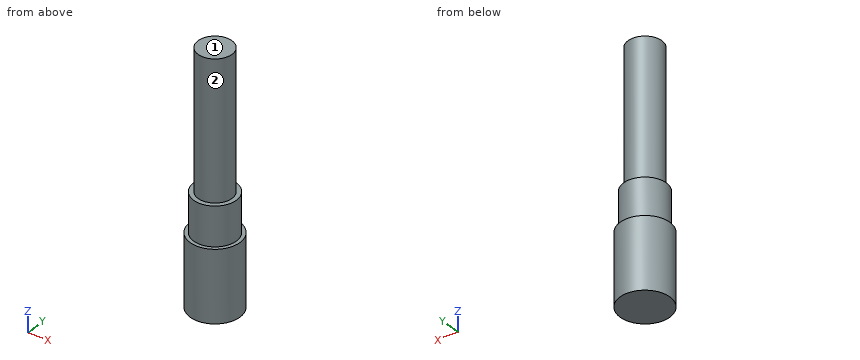
```python
from build123d import *

# Parameters (mm, degrees)
F0_R     = 15.38
F0_R_2   = 13.2
F1_DEPTH = 43.96
F0_R_3   = 10.45
F3_DEPTH = 68
F2_DEPTH = 152.8


with BuildPart() as f1:
    # F0 (on Top) → F1 (new body)
    with BuildSketch(Plane.XY):
        Circle(F0_R)
        Circle(F0_R_2, mode=Mode.SUBTRACT)
    extrude(amount=F1_DEPTH)

    # F0 (on Top) → F3 (join)
    with BuildSketch(Plane.XY):
        Circle(F0_R_2)
        Circle(F0_R_3, mode=Mode.SUBTRACT)
    extrude(amount=F3_DEPTH)

    # F0 (on Top) → F2 (join)
    with BuildSketch(Plane.XY):
        Circle(F0_R_3)
    extrude(amount=F2_DEPTH)


solid = f1.part
```
Geometry: final body of the model. Coordinates: model frame, mm. Face numbers are marked on the shaded views. A direction names the side the tool comes from. Round coordinates to 2 decimals unless told otherwise and drop trailing zeros. Order: outer loops, then holes, each group sorted by start corner. A loop starts at its lowest first (then second) coordinate and runs counter-clockwise, first axis right, second up. Notation, with made-up numbers: M 67.25,-16 L 125.25,-16 A21 cw 125.25,-3 Z; hole C -0.75,-16 d7. An arc over 180 degrees is marked long. Use one line per item in the form item = value. Start each with the question number.
Q1. Material intervals for line 1 (Z direction, x = 12.5, y = 7); line 2 (Z direction, x = -9, y = -8); line 3 (Y direction, x = 0.5, z = 86), sorted ascending. Write a range as [from, to].
Q2. Access query for the marked faces 1 and 2. Directions: +Z, -Z, +X, -X, +Y, -Y. A direction counts if a zero-diameter tool reaches every point of the face in a straight line with its end or side. Return the directions, or none.
Q3. Pin query (flat end, axial travel): pin 1 Ø1 at (y, z) = (9, 67) entering from -X; pin 2 Ø1 at (x, z) = (8, 98) entering from -Y; pin 3 Ø3 at (y, z) = (4.5, 123) entering from -X. Return the tip coordinate at first contact, or that it passes through.
Q4. Cut plane A-A (x = 0). Return loops of the section in (y, z).
Q5. Cut plane C-C (z = 125). Return loops of the section in (x, y).
Q6. Cut plane D-D (z = 19). Return loops of the section in (x, y), and give its area (3 significant figures).
Geometry results:
q1.line_1 = [0, 43.96]
q1.line_2 = [0, 68]
q1.line_3 = [-10.44, 10.44]
q2.face_1 = +Z, +X, -X, +Y, -Y
q2.face_2 = +Z
q3.pin_1 = -10.1
q3.pin_2 = -7.28
q3.pin_3 = -10.01
q4.outline = M -15.38,0 L 15.38,0 L 15.38,43.96 L 13.2,43.96 L 13.2,68 L 10.45,68 L 10.45,152.8 L -10.45,152.8 L -10.45,68 L -13.2,68 L -13.2,43.96 L -15.38,43.96 Z
q5.outline = C 0,0 d20.9
q6.outline = C 0,0 d30.76
q6.area = 743 mm^2
